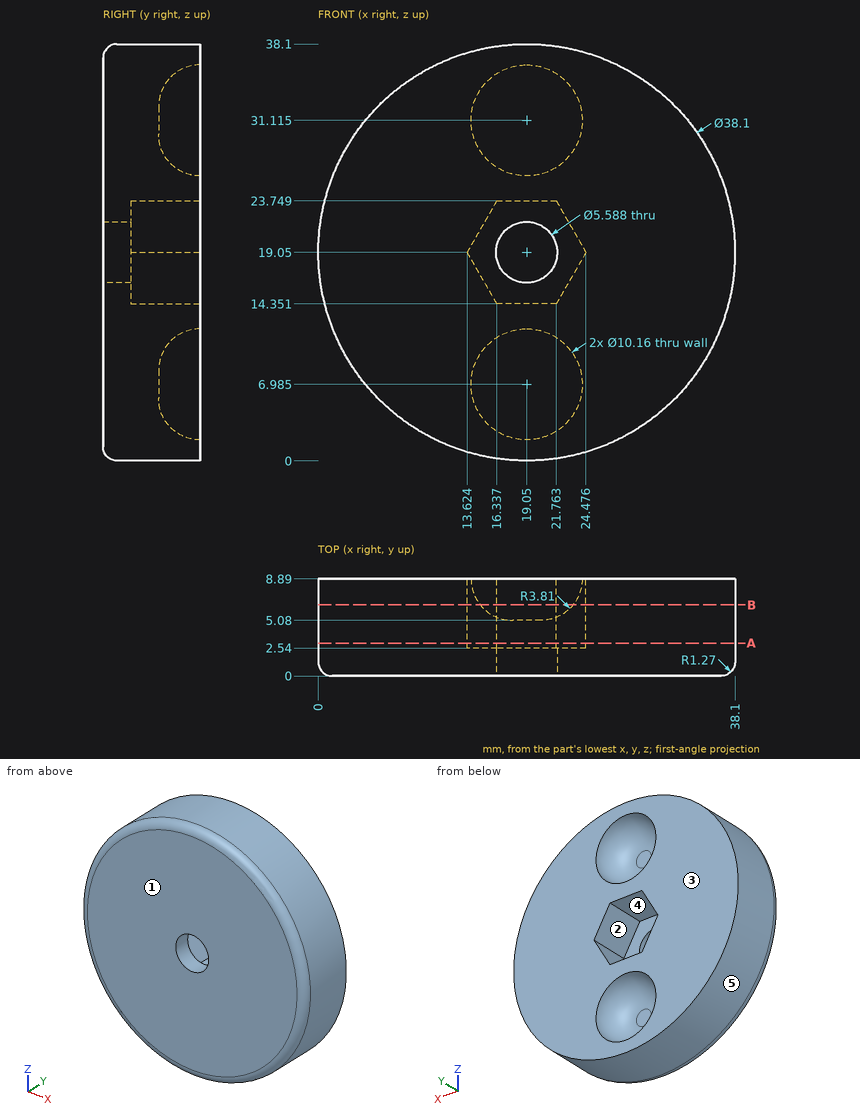
Print and shaded views of the part. All mm, measured from the part's lowest x, y and z. A direction names the side the tool comes from. Round coordinates to 2 decimals unless told otherwise and drop trailing zeros. Write each loop counter-clockwise with the first axis right and the second up, starting at its lowest first coordinate (ties: lowest second). Pieces come first, ordered by that corner, then holes.
Item 1: Drop flat-ended pins along their axis: pin 1 Ø2.5 at (x, y) = (20.5, 7) entering from +Z; pin 2 Ø1 at (x, y) = (26, 5) entering from -Z (3 decimals); pin 3 Ø3 at (y, z) = (7, 9) entering from -X. Give the stop position or say it passes through.
Results:
pin 1: stops at z = 38.1
pin 2: stops at z = 1.125
pin 3: stops at x = 2.03
Item 2: Two-plate mould, pull along X, no slides. Class the marked faces 3, 4 and 5: +X half, -X half, draft (parallel to the pull), parting line (faces both ways), or undercut.
Results:
face 3: draft
face 4: undercut
face 5: parting line
Item 3: Probe L1, parallel to X at y = 1.75, z = 19.05; L2, parallel to Z at x = 20.5, y = 8 (1 decimal); L3, parallel to X at y = 7, z = 27. List the from-to ranges inside material, lowest first.
Results:
L1: x = 0 to 16.26, 21.84 to 38.1
L2: z = 0.1 to 2.2, 11.7 to 14.4, 23.7 to 26.4, 35.9 to 38
L3: x = 1.74 to 17.04, 21.06 to 36.36
Item 4: Cut at B-B, the plane y = 6.5. Count the separate pieces of the cut face and the enclosed holes in it, plus the area to 3 significant figures.
Results:
separate pieces: 1
enclosed holes: 3
area: 951 mm2
Item 5: Cut at A-A, the plane y = 3. Give the cut face in (x, z), plus the area to 3 significant figures.
Results:
outline: circle Ø38.1 at (19.05, 19.05); hole (13.62, 19.05) - (16.34, 14.35) - (21.76, 14.35) - (24.48, 19.05) - (21.76, 23.75) - (16.34, 23.75) - close
area: 1,060 mm2
Item 6: Which spindle directions (+Z, -Z, +X, -X, +Y, -Y) get a long thin tool onto all of the face, cutting with end or side? Do the marked faces 1 and 2. Say none if no direction does.
Results:
face 1: +Z, -Z, +X, -X, -Y
face 2: +Y
